Input: part model. Units: mm. Frame: model coordinates. Round coordinates to 2 decimals unless told otherwise and drop trailing zeros. Use a Markdown table: item, result.
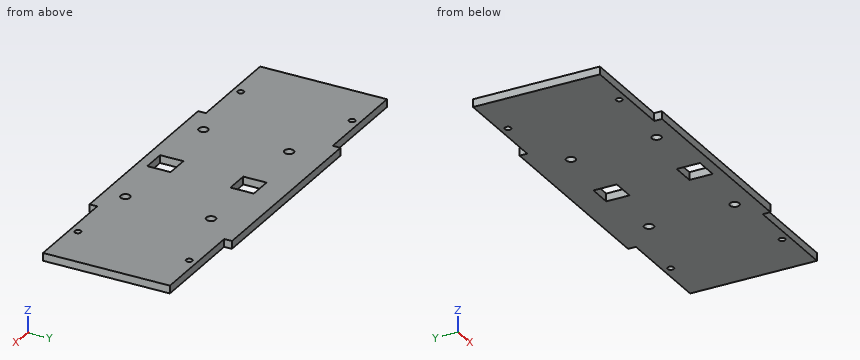
from build123d import *

# Parameters (mm, degrees)
SKETCH1_R           = 3
SKETCH1_W           = 15
SKETCH1_H           = 15
BOSS_EXTRUDE1_DEPTH = 5
SKETCH2_R           = 1.5
CUT_EXTRUDE1_DEPTH  = 185
SKETCH3_R           = 2
CUT_EXTRUDE2_DEPTH  = 10
SKETCH5_W           = 63.75
SKETCH5_H           = 5
BOSS_EXTRUDE3_DEPTH = 10
SKETCH6_W           = 127.5
SKETCH6_H           = 5
BOSS_EXTRUDE4_DEPTH = 10
SKETCH7_W           = 63.75
SKETCH7_H           = 5
BOSS_EXTRUDE5_DEPTH = 10
SKETCH8_R           = 2
BOSS_EXTRUDE6_DEPTH = 5
SKETCH8_3_R         = 2
CUT_EXTRUDE3_DEPTH  = 10


with BuildPart() as part:
    # Sketch1 → Boss-Extrude1 (new body)
    with BuildSketch(Plane.XY):
        Polygon((191.25, 71.637645579), (255, 71.637645579), (255, 0), (191.25, 0), (191.25, -5), (127.5, -5), (63.75, -5), (63.75, 0), (0, 0), (0, 71.637645579), (63.75, 71.637645579), (63.75, 76.637645579), (127.5, 76.637645579), (191.25, 76.637645579), align=None)
        with Locations((81.6684273, 63.35852795)):
            Circle(SKETCH1_R, mode=Mode.SUBTRACT)
        with Locations((173.3315727, 63.35852795)):
            Circle(SKETCH1_R, mode=Mode.SUBTRACT)
        with Locations((81.6684273, 8.27911763)):
            Circle(SKETCH1_R, mode=Mode.SUBTRACT)
        with Locations((173.3315727, 8.27911763)):
            Circle(SKETCH1_R, mode=Mode.SUBTRACT)
        with Locations((127.870410973, 62.57941032)):
            Rectangle(SKETCH1_W, SKETCH1_H, mode=Mode.SUBTRACT)
        with Locations((127.870410973, 9.058235259)):
            Rectangle(SKETCH1_W, SKETCH1_H, mode=Mode.SUBTRACT)
    extrude(amount=BOSS_EXTRUDE1_DEPTH)

    # Sketch2 → Cut-Extrude1 (cut)
    with BuildSketch(Plane(origin=(0, 0, 0), x_dir=(-1, 0, 0), z_dir=(0, 0, -1))):
        with Locations((-31.875, 5)):
            Circle(SKETCH2_R)
        with Locations((-31.875, 66.637645579)):
            Circle(SKETCH2_R)
        with Locations((-223.125, 66.637645579)):
            Circle(SKETCH2_R)
        with Locations((-223.125, 5)):
            Circle(SKETCH2_R)
    extrude(amount=-CUT_EXTRUDE1_DEPTH, mode=Mode.SUBTRACT)

    # Sketch3 → Cut-Extrude2 (cut)
    with BuildSketch(Plane(origin=(0, 0, 0), x_dir=(-1, 0, 0), z_dir=(0, 0, -1))):
        with Locations((-31.875, 5)):
            Circle(SKETCH3_R)
        with Locations((-31.875, 66.637645579)):
            Circle(SKETCH3_R)
        with Locations((-223.125, 5)):
            Circle(SKETCH3_R)
        with Locations((-223.125, 66.637645579)):
            Circle(SKETCH3_R)
    extrude(amount=-CUT_EXTRUDE2_DEPTH, mode=Mode.SUBTRACT)

    # Sketch5 → Boss-Extrude3 (add)
    with BuildSketch(Plane(origin=(0, 71.637645579, 0), x_dir=(1, 0, 0), z_dir=(0, 1, 0))):
        with Locations((223.125, -2.5)):
            Rectangle(SKETCH5_W, SKETCH5_H)
    extrude(amount=BOSS_EXTRUDE3_DEPTH)

    # Sketch6 → Boss-Extrude4 (add)
    with BuildSketch(Plane(origin=(0, 76.637645579, 0), x_dir=(1, 0, 0), z_dir=(0, 1, 0))):
        with Locations((127.5, -2.5)):
            Rectangle(SKETCH6_W, SKETCH6_H)
    extrude(amount=BOSS_EXTRUDE4_DEPTH)

    # Sketch7 → Boss-Extrude5 (add)
    with BuildSketch(Plane(origin=(0, 71.637645579, 0), x_dir=(1, 0, 0), z_dir=(0, 1, 0))):
        with Locations((31.875, -2.5)):
            Rectangle(SKETCH7_W, SKETCH7_H)
    extrude(amount=BOSS_EXTRUDE5_DEPTH)

    # Sketch8 → Boss-Extrude6 (add)
    with BuildSketch(Plane(origin=(0, 0, 0), x_dir=(-1, 0, 0), z_dir=(0, 0, -1))):
        with Locations((-31.875, 66.637645579)):
            Circle(SKETCH8_R)
        with Locations((-31.875, 76.637645579)):
            Circle(SKETCH8_R)
        with Locations((-223.125, 76.637645579)):
            Circle(SKETCH8_R)
        with Locations((-223.125, 66.637645579)):
            Circle(SKETCH8_R)
    extrude(amount=-BOSS_EXTRUDE6_DEPTH)

    # Sketch8<3> → Cut-Extrude3 (cut)
    with BuildSketch(Plane(origin=(0, 0, 0), x_dir=(-1, 0, 0), z_dir=(0, 0, -1))):
        with Locations((-31.875, 76.637645579)):
            Circle(SKETCH8_3_R)
        with Locations((-223.125, 76.637645579)):
            Circle(SKETCH8_3_R)
    extrude(amount=-CUT_EXTRUDE3_DEPTH, mode=Mode.SUBTRACT)


solid = part.part
1) Contact query for flat-ended pins moving along their axis: P1, Ø5, axis at x = 173.33, y = 8.28, coming from the +Z side; P2, Ø1.5, axis at y = 85, z = 2.5, coming from the -X side. Output: stop coordinate, or through.
Answer key:
| item | result |
|---|---|
| P1 | passes through |
| P2 | stops at x = 63.75 |
2) Cut plane A-A on z = 3.45. State how many separate pieces and enclosed holes the cut face has, and give its area (3 significant figures).
Answer key:
| item | result |
|---|---|
| separate pieces | 1 |
| enclosed holes | 10 |
| area | 21,500 mm^2 |
3) Ray query, probe 1 along X at (y, z) = (59.5, 2.5); probe 2 along X at (y, z) = (65, 0.8); probe 3 along X at (y, z) = (66, 0.3). Return the intervals inside material, ascending.
Answer key:
| item | result |
|---|---|
| probe 1 | x = 0 to 120.37, 135.37 to 255 |
| probe 2 | x = 0 to 79.16, 84.18 to 120.37, 135.37 to 170.82, 175.84 to 255 |
| probe 3 | x = 0 to 80.25, 83.09 to 120.37, 135.37 to 171.91, 174.75 to 255 |
